Autodesk Inventor part; units mm, degrees
ref_plane "YZ Plane" through (0, 0, 0) normal (1, 0, 0) x (0, 1, 0)
ref_plane "XZ Plane" through (0, 0, 0) normal (0, 1, 0) x (-1, 0, 0)
ref_plane "XY Plane" through (0, 0, 0) normal (0, 0, 1) x (1, 0, 0)
sketch "Эскиз1" plane through (0, 0, 0) normal (0, 0, 1) x (1, 0, 0)
  circle A0 centre (0, 0) radius 10
  line L0 (0, 0) -> (-6.25, 0) construction
  line L1 (0, 0) -> (6.25, 0) construction
  circle A1 centre (-6.25, 0) radius 1.5
  circle A2 centre (6.25, 0) radius 1.5
  circle A3 centre (0, -6.25) radius 1.5
  circle A4 centre (0, 6.25) radius 1.5
  line L2 (0, 0) -> (0, -6.25) construction
  line L3 (0, 0) -> (0, 6.25) construction
  arc A5 (1.3229, -1.5) -> (-1.3229, -1.5) centre (0, 0) ccw
  line L4 (0, 0) -> (0, -1.5) construction
  line L5 (1.3229, -1.5) -> (-1.3229, -1.5)
  dimension "d0" = 20
  dimension "d1" = 6.25
  dimension "d2" = 6.25
  dimension "d3" = 3
  dimension "d4" = 3
  dimension "d7" = 90
  dimension "d9" = 4
  dimension "d10" = 1.5
extrude "Выдавливание1" add sketch "Эскиз1" along normal blind 7
properties part number "sleeve for kick"
Input: part model. Units: mm. Frame: model coordinates. A direction names the side the tool comes from. Give positions to 0.01 mm unless a question says otherwise; leave off trailing zeros. Order: outer loops, then holes, each group sorted by start corner. A loop starts at its lowest first (then second) coordinate and runs counter-clockwise, first axis right, second up. Notation, with made-up numbers: M 34,77.25 L 64,77.25 A21 ccw 64,105.25 Z; hole C 34.25,88 d4. An arc over 180 degrees is marked long. Answer as a JSON object with one key per item and string values.
1. First-contact query: P1, Ø1, axis at x = -3.5, z = 3, coming from the +Y side; P2, Ø2.5, axis at x = 0, y = 0, coming from the -Z side; P3, Ø4, axis at x = 2.5, z = 1.5, coming from the +Y side; P4, Ø4, axis at x = 0, y = -6.25, coming from the +Z side. Flat tips, straight axial feed; report the tip coordinate or a pass-through.
Result sheet:
{"P1": "y = 9.54", "P2": "through", "P3": "y = 9.99", "P4": "z = 7"}
2. Cut plane D-D, the plane x = 7.25. Output: boundary loops of the cut face in (y, z).
Result sheet:
{"outline": "M -6.89,0 L -1.12,0 L -1.12,7 L -6.89,7 Z; M 1.12,0 L 6.89,0 L 6.89,7 L 1.12,7 Z"}
3. Reachability of faces 4 (the flat face through (0, -1.5, 3)), 5 (the flat face through (0, -2, 0)) from +Z, -Z, +X, -X, +Y, -Y: full face, straight path, thin tool, end or side. Return the list, or none.
Result sheet:
{"face 4": "+Z, -Z", "face 5": "-Z, +X, -X, +Y, -Y"}
4. Cut plane A-A, the plane x = 0. Output: boundary loops of the cut face in (y, z), and give its area (3 significant figures).
Result sheet:
{"outline": "M -10,0 L -7.75,0 L -7.75,7 L -10,7 Z; M -4.75,0 L -1.5,0 L -1.5,7 L -4.75,7 Z; M 2,0 L 4.75,0 L 4.75,7 L 2,7 Z; M 7.75,0 L 10,0 L 10,7 L 7.75,7 Z", "area": "73.5 mm²"}
5. Pull-direction query (Y, two-part tool) for faces 1 (the cylindrical face through (-2.17, 9.76, 3.45)), 2 (the flat face through (0, -2, 7)), 3 (the cylindrical face through (0, 2, 3)); classes: +Y half, -Y half, draft (parallel to the pull), parting line (faces both ways), or undercut.
Result sheet:
{"face 1": "parting line", "face 2": "draft", "face 3": "undercut"}
6. Cut plane C-C, the plane y = 1. Output: boundary loops of the cut face in (x, z), and give its area (3 significant figures).
Result sheet:
{"outline": "M -9.95,0 L -7.37,0 L -7.37,7 L -9.95,7 Z; M -5.13,0 L -1.73,0 L -1.73,7 L -5.13,7 Z; M 1.73,0 L 5.13,0 L 5.13,7 L 1.73,7 Z; M 7.37,0 L 9.95,0 L 9.95,7 L 7.37,7 Z", "area": "83.7 mm²"}
7. Ray query, line 1 (Y direction, x = 0, z = 1.5); line 2 (X direction, y = -1, z = 5); line 3 (Y direction, x = 6.25, z = 4). Return the intervals inside material, ascending. Write a range as [from, to].
Result sheet:
{"line 1": "[-10, -7.75], [-4.75, -1.5], [2, 4.75], [7.75, 10]", "line 2": "[-9.95, -7.37], [-5.13, -1.73], [1.73, 5.13], [7.37, 9.95]", "line 3": "[-7.81, -1.5], [1.5, 7.81]"}
8. Cut plane B-B, the plane z = 6.5. Output: boundary loops of the cut face in (x, y).
Result sheet:
{"outline": "C 0,0 d20; hole C -6.25,0 d3; hole C 0,-6.25 d3; hole C 0,6.25 d3; hole M -1.32,-1.5 L 1.32,-1.5 A2 ccw long Z; hole C 6.25,0 d3"}
